```python
from build123d import *

# Parameters (mm, degrees)
SKETCH_4_W = 1
SKETCH_4_H = 1


with BuildPart() as part:
    # 草图1 → 旋转1 (revolve)
    with BuildSketch(Plane(origin=(0, 0, 0), x_dir=(0, 0, -1), z_dir=(1, 0, 0))):
        Polygon((0, 63), (4, 63), (4, 62), (3, 62), (3, 0), (0, 0), align=None)
    revolve(axis=Axis((0, 0, 0), (0, 1, 0)))

    # 草图4 → 切除-旋转1 (revolve, cut)
    with BuildSketch(Plane.XY, mode=Mode.PRIVATE) as cut_revolve_1_sk:
        with Locations((2.5, 1.5)):
            Rectangle(SKETCH_4_W, SKETCH_4_H)
    revolve(cut_revolve_1_sk.sketch.rotate(Axis((0, 0, 0), (0, 1, 0)), 90), axis=Axis((0, 0, 0), (0, 1, 0)), mode=Mode.SUBTRACT)


solid = part.part
```
Source: CAD feature listing. Evaluate the final solid. Frame: model axes, mm. A direction names the side the tool comes from. Round coordinates to 2 decimals unless told otherwise and drop trailing zeros. Loops run counter-clockwise (first coordinate to the right, second up) from the corner with the lowest first, then second, coordinate; pieces in that order, holes last.
1. Section query A-A on x = 0. Output: boundary loops of the cut face in (y, z), and give its area (3 significant figures).
2. Section query B-B on z = 0.75. Output: boundary loops of the cut face in (x, y).
3. Mould query, pull axis Y, two halves, no side actions, for faces 4 (the flat face through (0, 63, 0)), 5 (the cylindrical face through (-0.1, 0.5, 3)), 6 (the cylindrical face through (1.952, 1.507, 0.434)), 7 (the flat face through (0, 0, 0)). Classes: released by +Y, released by -Y, zero draft, split by the parting line, or undercut.
4. Access query for faces 1 (the cylindrical face through (3.905, 62.493, 0.867)), 2 (the flat face through (2, 2, 1)), 3 (the flat face through (-3, 62, -1)). Directions: +Z, -Z, +X, -X, +Y, -Y. A direction counts if a zero-diameter tool reaches every point of the face in a straight line with its end or side. Return the directions, or none.
5. Ray query, L1, parallel to Y at x = 1, z = 2.5; L2, parallel to X at y = 11.5, z = 0; L3, parallel to Y at x = 3.5, z = -0.25. Return the intervals inside material, ascending.
6. Contact query for flat-ended pins moving along their axis: pin 1 (4 mm diameter, centred on y = 23.5, z = -0.5, fed in from -X); pin 2 (3 mm diameter, centred on y = 7.5, z = 2.5, fed in from -X); pin 3 (1 mm diameter, centred on x = -0.5, y = 52, fed in from +Z). Output: stop coordinate, or through.
7. Section query C-C on y = 33.5. Output: boundary loops of the cut face in (x, z), and give its area (3 significant figures).
Answers below:
1. outline: (0, -3) - (1, -3) - (1, -2) - (2, -2) - (2, -3) - (62, -3) - (62, -4) - (63, -4) - (63, 4) - (62, 4) - (62, 3) - (2, 3) - (2, 2) - (1, 2) - (1, 3) - (0, 3) - close
1. area: 378 mm2
2. outline: (-3.93, 62) - (-2.9, 62) - (-2.9, 2) - (-1.85, 2) - (-1.85, 1) - (-2.9, 1) - (-2.9, 0) - (2.9, 0) - (2.9, 1) - (1.85, 1) - (1.85, 2) - (2.9, 2) - (2.9, 62) - (3.93, 62) - (3.93, 63) - (-3.93, 63) - close
3. face 4: released by +Y
3. face 5: zero draft
3. face 6: undercut
3. face 7: released by -Y
4. face 1: +Y, -Y
4. face 2: none
4. face 3: -Y
5. L1: y = 0 to 1, 2 to 63
5. L2: x = -3 to 3
5. L3: y = 62 to 63
6. pin 1: stops at x = -3
6. pin 2: stops at x = -2.83
6. pin 3: stops at z = 3
7. outline: circle Ø6 at (0, 0)
7. area: 28.3 mm2
